Build history of the part. All positions in model axes, mm. A direction names the side the tool comes from. Round coordinates to 2 decimals unless told otherwise and drop trailing zeros. Write each loop counter-clockwise with the first axis right and the second up, starting at its lowest first coordinate (ties: lowest second). Pieces come first, ordered by that corner, then holes. Notation, with made-up numbers: (61.5, 67) - (76.5, 67) arc R22 ccw to (76.5, 98) - close; hole circle Ø9 at (75, -34.75). An arc over 180 degrees is marked (long way). Write each question's results on one line, items separated by ' | '.
Autodesk Inventor part; units mm, degrees
ref_plane "YZ Plane" through (0, 0, 0) normal (1, 0, 0) x (0, 1, 0)
ref_plane "XZ Plane" through (0, 0, 0) normal (0, 1, 0) x (-1, 0, 0)
ref_plane "XY Plane" through (0, 0, 0) normal (0, 0, 1) x (1, 0, 0)
sketch "Sketch1" plane through (0, 0, 0) normal (0, 0, 1) x (1, 0, 0)
  line L0 (0, 0) -> (184.15, 0)
  line L1 (184.15, 0) -> (184.15, -107.95)
  line L2 (184.15, -107.95) -> (0, -107.95)
  line L3 (0, -107.95) -> (0, 0)
  dimension "d0" = 107.95
  dimension "d1" = 184.15
extrude "Extrusion1" add sketch "Sketch1" along normal blind 177.8
sketch "Sketch2" plane through (0, 0, 177.8) normal (0, 0, 1) x (1, 0, 0)
  line L0 (0, 0) -> (0, -107.95)
  line L1 (184.15, -107.95) -> (184.15, 0)
  line L2 (0, -76.2) -> (184.15, -76.2)
  line L3 (184.15, -76.2) -> (184.15, -82.55)
  line L4 (184.15, -82.55) -> (0, -82.55)
  line L5 (0, -82.55) -> (0, -76.2)
  line L6 (0, -107.95) -> (184.15, -107.95)
  dimension "d4" = 6.35
  dimension "d5" = 25.4
extrude "Extrusion2" add sketch "Sketch2" along normal blind 19.05 contours L2 L1 L4 L0
sketch "Sketch3" plane through (0, 0, 0) normal (0, 0, -1) x (-1, 0, 0)
  line L0 (0, -107.95) -> (0, 0)
  line L1 (-184.2181, -76.2) -> (0, -76.2)
  line L2 (0, -76.2) -> (0, -82.55)
  line L3 (0, -82.55) -> (-184.2181, -82.55)
  line L4 (-184.2181, -82.55) -> (-184.2181, -76.2)
  line L5 (-184.15, -107.95) -> (0, -107.95)
  line L6 (0, 0) -> (-184.15, 0)
  dimension "d8" = 25.4
  dimension "d9" = 76.2
extrude "Extrusion3" add sketch "Sketch3" along normal blind 19.05
sketch "Sketch4" plane through (184.15, 0, 177.8) normal (1, 0, 0) x (0, 0, -1)
  line L0 (177.8, -76.2) -> (177.8, -82.55)
  line L1 (177.8, -76.2) -> (196.85, -76.2)
  point P0 (177.8, 0)
  point P1 (0, -82.55)
  point P2 (0, -76.2)
sketch "Sketch5" plane through (184.15, 0, 177.8) normal (1, 0, 0) x (0, 0, -1)
  point P0 (177.8, 0)
sketch "Sketch6" plane through (0, 0, 0) normal (0, 0, -1) x (-1, 0, 0)
  line L0 (-181.61, -2.54) -> (-2.54, -2.54)
  line L1 (-2.54, -2.54) -> (-2.54, -76.2)
  line L2 (-2.54, -76.2) -> (-181.61, -76.2)
  line L3 (-181.61, -76.2) -> (-181.61, -2.54)
  line L4 (0, 0) -> (-184.15, 0)
  line L5 (0, -76.2) -> (0, 0)
  line L6 (-184.15, 0) -> (-184.15, -76.2)
  line L7 (0, -76.2) -> (-184.2181, -76.2)
  dimension "d12" = 2.54
  dimension "d13" = 2.54
  dimension "d14" = 2.54
  dimension "d15" = 0
extrude "Extrusion4" cut sketch "Sketch6" against normal blind 175.26 contours L0 L1 L2 L3
sketch "Sketch7" plane through (0, 0, 0) normal (0, 0, -1) x (-1, 0, 0)
  point P0 (0, 0)
sketch "Sketch8" plane through (0, 0, 0) normal (0, 0, -1) x (-1, 0, 0)
  line L0 (0, -82.55) -> (-184.15, -82.55)
  line L1 (-184.15, -82.55) -> (-184.15, -107.95)
  line L2 (-184.15, -107.95) -> (0, -107.95)
  line L3 (0, -107.95) -> (0, -82.55)
  point P0 (0, 0)
extrude "Extrusion5" cut sketch "Sketch8" against normal blind 177.8
properties part number "robotics battery box"
(1) Slice it at B-B, the plane y = -27. Write the cut outline in (x, z).
Worked answers:
outline: (0, 0) - (2.54, 0) - (2.54, 175.26) - (181.61, 175.26) - (181.61, 0) - (184.15, 0) - (184.15, 177.8) - (0, 177.8) - close
(2) Slice it at D-D, the plane z = -5.5. Write the cut outline in (x, y), and give its area (3 significant figures).
Worked answers:
outline: (0, -82.55) - (184.22, -82.55) - (184.22, -76.2) - (0, -76.2) - close | area: 1,170 mm2
(3) Flat gauge pins, fed straight in: pin 1 Ø1 at (x, y) = (88.5, -40.5) entering from -Z; pin 2 Ø1 at (y, z) = (-69.5, 68.5) entering from +X; pin 3 Ø2 at (x, y) = (53.5, -21.5) entering from +Z. Where does each tip first touch, or does it go through?
Worked answers:
pin 1: stops at z = 175.26 | pin 2: stops at x = 184.15 | pin 3: stops at z = 177.8
(4) Slice it at C-C, the plane x = 30. Write the cut outline in (y, z), and give its area (3 significant figures).
Worked answers:
outline: (-82.55, -19.05) - (-76.2, -19.05) - (-76.2, 175.26) - (-2.54, 175.26) - (-2.54, 0) - (0, 0) - (0, 177.8) - (-76.2, 177.8) - (-76.2, 196.85) - (-82.55, 196.85) - close | area: 2,010 mm2
(5) Drill centre lines: probe 1 along X at (y, z) = (-20.5, 17); probe 2 along Y at (x, z) = (43.5, 48); probe 3 along Z at (x, y) = (26, -12.5). Where is each one in solid material? Low to high. Write a range as [from, to].
Worked answers:
probe 1: x = [0, 2.54], [181.61, 184.15] | probe 2: y = [-82.55, -76.2], [-2.54, 0] | probe 3: z = [175.26, 177.8]
(6) Two-plate mould, pull along X, no slides. Class faces 5 (the flat face through (91, -79, 196.85)), 6 (the flat face through (93, -39, 175.26)), 7 (the flat face through (184.218, -79, -9)), 8 (the flat face through (2.54, -39, 86)): released by +X, released by -X, zero draft, split by the parting line, or undercut.
Worked answers:
face 5: zero draft | face 6: undercut | face 7: released by +X | face 8: undercut
(7) Tool access for faces 1 (the flat face through (92, -1, 0)), 2 (the flat face through (93, -76.2, 79)), 3 (the flat face through (91, -76.2, 187)), 4 (the flat face through (93, -79, -19.05)): list every direction of +Z, -Z, +X, -X, +Y, -Y with a clear straight run to the whole face (end or side of a thin tool).
Worked answers:
face 1: -Z, +X, -X, +Y | face 2: -Z | face 3: +Z, +X, -X, +Y | face 4: -Z, +X, -X, +Y, -Y
(8) Slice it at A-A, the plane z = 114.5. Write the cut outline in (x, y).
Worked answers:
outline: (0, -82.55) - (184.15, -82.55) - (184.15, 0) - (0, 0) - close; hole (2.54, -76.2) - (181.61, -76.2) - (181.61, -2.54) - (2.54, -2.54) - close
